For this review, take the finished solid that the model builds, in its own axes (mm). A direction names the side the tool comes from. Coordinates: 2 decimals unless noted, no trailing zeros. Write each loop counter-clockwise with the first axis right and the second up, starting at its lowest first coordinate (ties: lowest second). Pieces come first, ordered by that corner, then holes.
```python
from build123d import *

# Parameters (mm, degrees)
SKETCH1_W           = 61
SKETCH1_H           = 44
SKETCH1_W_2         = 55
SKETCH1_H_2         = 38
BOSS_EXTRUDE1_DEPTH = 23
SKETCH2_W           = 61
SKETCH2_H           = 44
BOSS_EXTRUDE2_DEPTH = 2.3
SKETCH3_W           = 2.5
SKETCH3_H           = 44
BOSS_EXTRUDE3_DEPTH = 23
SKETCH5_W           = 2.5
SKETCH5_H           = 44
BOSS_EXTRUDE4_DEPTH = 23
SKETCH6_R           = 1.5
CUT_EXTRUDE1_DEPTH  = 23


with BuildPart() as part:
    # Sketch1 → Boss-Extrude1 (new body)
    with BuildSketch(Plane.XY):
        Rectangle(SKETCH1_W, SKETCH1_H)
        Rectangle(SKETCH1_W_2, SKETCH1_H_2, mode=Mode.SUBTRACT)
    extrude(amount=BOSS_EXTRUDE1_DEPTH)

    # Sketch2 → Boss-Extrude2 (add)
    with BuildSketch(Plane.XY.offset(23)):
        Rectangle(SKETCH2_W, SKETCH2_H)
    extrude(amount=BOSS_EXTRUDE2_DEPTH)

    # Sketch3 → Boss-Extrude3 (add)
    with BuildSketch(Plane.ZY.offset(30.5)):
        with Locations((1.25, 0)):
            Rectangle(SKETCH3_W, SKETCH3_H)
    extrude(amount=BOSS_EXTRUDE3_DEPTH)

    # Sketch5 → Boss-Extrude4 (add)
    with BuildSketch(Plane(origin=(30.5, 0, 0), x_dir=(0, 0, -1), z_dir=(1, 0, 0))):
        with Locations((-1.25, 0)):
            Rectangle(SKETCH5_W, SKETCH5_H)
    extrude(amount=BOSS_EXTRUDE4_DEPTH)

    # Sketch6 → Cut-Extrude1 (cut)
    with BuildSketch(Plane.XY.offset(2.5)):
        with Locations((42, 11)):
            Circle(SKETCH6_R)
        with Locations(Location((42, -11, 0), (0, 0, 180))):
            Circle(SKETCH6_R)
        with Locations((-42, -11)):
            Circle(SKETCH6_R)
        with Locations(Location((-42, 11, 0), (0, 0, 180))):
            Circle(SKETCH6_R)
    extrude(amount=-CUT_EXTRUDE1_DEPTH, mode=Mode.SUBTRACT)


solid = part.part
```
Q1. Add section A-A (y = -11). State the section outline as (x, z) points, then the cut area to 3 significant figures.
Ans:
outline: (-53.5, 0) - (-43.5, 0) - (-43.5, 2.5) - (-53.5, 2.5) - close; (-40.5, 0) - (-27.5, 0) - (-27.5, 23) - (27.5, 23) - (27.5, 0) - (40.5, 0) - (40.5, 2.5) - (30.5, 2.5) - (30.5, 25.3) - (-30.5, 25.3) - (-30.5, 2.5) - (-40.5, 2.5) - close; (43.5, 0) - (53.5, 0) - (53.5, 2.5) - (43.5, 2.5) - close
area: 378 mm2
Q2. Add section C-C (z = 13.75). State the section outline as (x, y) points, then the cut area to 3 significant figures.
Ans:
outline: (-30.5, -22) - (30.5, -22) - (30.5, 22) - (-30.5, 22) - close; hole (-27.5, -19) - (27.5, -19) - (27.5, 19) - (-27.5, 19) - close
area: 594 mm2
Q3. Add section B-B (x = -42). State the section outline as (y, z) points.
Ans:
outline: (-22, 0) - (-12.5, 0) - (-12.5, 2.5) - (-22, 2.5) - close; (-9.5, 0) - (9.5, 0) - (9.5, 2.5) - (-9.5, 2.5) - close; (12.5, 0) - (22, 0) - (22, 2.5) - (12.5, 2.5) - close
Q4. Tool access review of faces 1 (the flat face through (30.5, 0, 14)), 2 (the flat face through (-42, 0, 2.5)), 3 (the flat face through (0, 19, 11)): name each direction out of +Z, -Z, +X, -X, +Y, -Y from which nothing blocks a thin tool from reaching the whole face with its end or side.
Ans:
face 1: +Z, +X, +Y, -Y
face 2: +Z, -X, +Y, -Y
face 3: -Z
Q5. Clearance check with flat-ended pins moving along their axes: pin 1 Ø3 at (y, z) = (16, 15) entering from -X; pin 2 Ø4 at (y, z) = (1, 18) entering from +X; pin 3 Ø1.5 at (x, y) = (5.5, 0.5) entering from -Z. State where each tip first meets the part, or that it passes through.
Ans:
pin 1: stops at x = -30.5
pin 2: stops at x = 30.5
pin 3: stops at z = 23
Q6. Add section D-D (x = 8.5). State the section outline as (y, z) points.
Ans:
outline: (-22, 0) - (-19, 0) - (-19, 23) - (19, 23) - (19, 0) - (22, 0) - (22, 25.3) - (-22, 25.3) - close
Q7. For probe 1 along Y at (x, z) = (42, 0.6); probe 2 along X at (y, z) = (4.5, 11.25); probe 3 along X at (y, z) = (18.5, 1), list the stretches that pass through material, from the lowest coordinate up.
Ans:
probe 1: y = -22 to -12.5, -9.5 to 9.5, 12.5 to 22
probe 2: x = -30.5 to -27.5, 27.5 to 30.5
probe 3: x = -53.5 to -27.5, 27.5 to 53.5
Q8. Draft analysis for pull direction Y (two halves, no side actions). For faces 4 (the flat face through (-30.5, 0, 14)), 5 (the flat face through (-1, 22, 13)), 6 (the flat face through (-1, -22, 13)), 7 (the cylindrical face through (40.5, 11.07, 1.27)), state which applies: +Y half, -Y half, draft (parallel to the pull), parting line (faces both ways), or undercut.
Ans:
face 4: draft
face 5: +Y half
face 6: -Y half
face 7: undercut
